Could you check a few things on this model? Use its own coordinates, in mm. Face numbers are marked on the shaded views. Give positions to 0.01 mm unless a question says otherwise; leave off trailing zeros. Loops run counter-clockwise (first coordinate to the right, second up) from the corner with the lowest first, then second, coordinate; pieces in that order, holes last. Notation, with made-up numbers: (58.5, -7) - (89.5, -7) arc R12 ccw to (89.5, -3) - close; hole circle Ø7 at (-21, -13.5). An arc over 180 degrees is marked (long way). Write each question's results on one line, items separated by ' | '. Start each with the question number.
1) I want a section at A-A, the plane x = 6. Write out the boundary of the cut face in (y, z), and give its area (3 significant figures).
2) If we mould it in two halves opening along Z, with no side actions, what happens to the marked faces 1 and 2? For each: +Z half, -Z half, draft (parallel to the pull), parting line (faces both ways), or undercut.
3) I want a section at B-B, the plane z = 66. Write out the boundary of the cut face in (x, y), and give its area (3 significant figures).
4) I want a section at D-D, the plane y = 9. Count the separate pieces of the cut face and the enclosed holes in it, and give its area (3 significant figures).
5) I want a section at C-C, the plane x = 34. Write out the boundary of the cut face in (y, z), and give its area (3 significant figures).
6) I'm going to push flat-ended pins straight in: pin 1 (1 mm diameter, centred on x = 42.5, z = 4, fed in from +Y); pin 2 (3.5 mm diameter, centred on x = -54.46, z = 79.5, fed in from +Y); pin 3 (6.5 mm diameter, centred on x = -54.5, z = -80, fed in from -Y). Where does each tip first touch, or does it pass through?
7) If I drill on probe 1 along Z at (x, y) = (23, 13.75); probe 2 along X at (y, z) = (4.5, 15.5); probe 3 along Y at (x, z) = (-14.5, 73), over which ranges is the centre line in solid material (lowest first)? Write a range as [from, to].
from build123d import *

# Parameters (mm, degrees)
BOSS_EXTRUDE1_DEPTH                                 = 15.0114
CUT_EXTRUDE1_DEPTH                                  = 11.9634
MIRROR2_COPY_1_DEPTH                                = 11.9634
CBORE_SLOT_FOR_3_BINDING_HEAD_MACHINE_S_D           = 4.3688
CBORE_SLOT_FOR_3_BINDING_HEAD_MACHINE_S_CBORE_D     = 7.874
CBORE_SLOT_FOR_3_BINDING_HEAD_MACHINE_S_CBORE_DEPTH = 3.048
MIRROR4_COPY_1_D                                    = 4.3688
MIRROR4_COPY_1_CBORE_D                              = 7.874
MIRROR4_COPY_1_CBORE_DEPTH                          = 3.048
SKETCH10_W                                          = 20.32
SKETCH10_H                                          = 20.32
CUT_EXTRUDE3_DEPTH                                  = 3.048


with BuildPart() as part:
    # Sketch2 → Boss-Extrude1 (new body)
    with BuildSketch(Plane(origin=(0, 0, 0), x_dir=(1, 0, 0), z_dir=(0, 1, 0))):
        with BuildLine():
            Line((56.6928, -85.4964), (-56.6928, -85.4964))
            ThreePointArc((-56.6928, -85.4964), (-59.386876836, -84.380476836), (-60.5028, -81.6864))
            Line((-60.5028, -81.6864), (-60.5028, 81.6864))
            ThreePointArc((-60.5028, 81.6864), (-59.386876836, 84.380476836), (-56.6928, 85.4964))
            Line((-56.6928, 85.4964), (56.6928, 85.4964))
            ThreePointArc((56.6928, 85.4964), (59.386876836, 84.380476836), (60.5028, 81.6864))
            Line((60.5028, 81.6864), (60.5028, -81.6864))
            ThreePointArc((60.5028, -81.6864), (59.386876836, -84.380476836), (56.6928, -85.4964))
        make_face()
    extrude(amount=BOSS_EXTRUDE1_DEPTH)

    # Sketch3 → Cut-Extrude1 (cut)
    with BuildSketch(Plane(origin=(0, 15.0114, 0), x_dir=(1, 0, 0), z_dir=(0, 1, 0))):
        with BuildLine():
            Line((-55.9054, 0), (-55.9054, 71.294481899))
            ThreePointArc((-55.9054, 71.294481899), (-55.361345544, 72.607945544), (-54.047881899, 73.152))
            Line((-54.047881899, 73.152), (-47.553880656, 73.152))
            ThreePointArc((-47.553880656, 73.152), (-44.550315934, 74.249721203), (-42.962410096, 77.0255))
            ThreePointArc((-42.962410096, 77.0255), (-41.374504259, 79.801278797), (-38.370939537, 80.899))
            Line((-38.370939537, 80.899), (0, 80.899))
            Line((0, 80.899), (0, 0))
            Line((0, 0), (-55.9054, 0))
        make_face()
    cut_extrude1 = extrude(amount=-CUT_EXTRUDE1_DEPTH, mode=Mode.SUBTRACT)

    # Mirror1: Cut-Extrude1 across plane
    add(cut_extrude1.mirror(Plane(origin=(0, 0, 0), x_dir=(0, 0, 1), z_dir=(1, 0, 0))), mode=Mode.SUBTRACT)

    # Mirror2: Cut-Extrude1 across plane
    add(cut_extrude1.mirror(Plane.XY), mode=Mode.SUBTRACT)

    # Mirror2 copy 1 sketch → Mirror2 copy 1 (cut)
    with BuildSketch(Plane(origin=(0, 15.0114, 0), x_dir=(-1, 0, 0), z_dir=(0, 1, 0))):
        with BuildLine():
            Line((-55.9054, 0), (-55.9054, 71.294481899))
            ThreePointArc((-55.9054, 71.294481899), (-55.361345544, 72.607945544), (-54.047881899, 73.152))
            Line((-54.047881899, 73.152), (-47.553880656, 73.152))
            ThreePointArc((-47.553880656, 73.152), (-44.550315934, 74.249721203), (-42.962410096, 77.0255))
            ThreePointArc((-42.962410096, 77.0255), (-41.374504259, 79.801278797), (-38.370939537, 80.899))
            Line((-38.370939537, 80.899), (0, 80.899))
            Line((0, 80.899), (0, 0))
            Line((0, 0), (-55.9054, 0))
        make_face()
    extrude(amount=-MIRROR2_COPY_1_DEPTH, mode=Mode.SUBTRACT)

    # CBORE SLOT for #3 Binding Head Machine Screw1 (through all)
    with Locations(Plane(origin=(0, 0, 0), x_dir=(-1, 0, 0), z_dir=(0, -1, 0))):
        with Locations((-54.4576, 79.502)):
            cbore_slot_for_3_binding_head_machine_s = CounterBoreHole(CBORE_SLOT_FOR_3_BINDING_HEAD_MACHINE_S_D / 2, CBORE_SLOT_FOR_3_BINDING_HEAD_MACHINE_S_CBORE_D / 2, CBORE_SLOT_FOR_3_BINDING_HEAD_MACHINE_S_CBORE_DEPTH)

    # Mirror3: CBORE SLOT for #3 Binding Head Machine Screw1 across plane
    add(cbore_slot_for_3_binding_head_machine_s.mirror(Plane(origin=(0, 0, 0), x_dir=(0, 0, 1), z_dir=(1, 0, 0))), mode=Mode.SUBTRACT)

    # Mirror4: CBORE SLOT for #3 Binding Head Machine Screw1 across plane
    add(cbore_slot_for_3_binding_head_machine_s.mirror(Plane.XY), mode=Mode.SUBTRACT)

    # Mirror4 copy 1 (through all)
    with Locations(Plane.XZ):
        with Locations((-54.4576, 79.502)):
            CounterBoreHole(MIRROR4_COPY_1_D / 2, MIRROR4_COPY_1_CBORE_D / 2, MIRROR4_COPY_1_CBORE_DEPTH)

    # Sketch10 → Cut-Extrude3 (cut)
    with BuildSketch(Plane.XZ):
        with Locations((0, 67.66)):
            Rectangle(SKETCH10_W, SKETCH10_H)
    cut_extrude3 = extrude(amount=-CUT_EXTRUDE3_DEPTH, mode=Mode.SUBTRACT)

    # Mirror7: Cut-Extrude3 across plane
    add(cut_extrude3.mirror(Plane.XY), mode=Mode.SUBTRACT)


solid = part.part
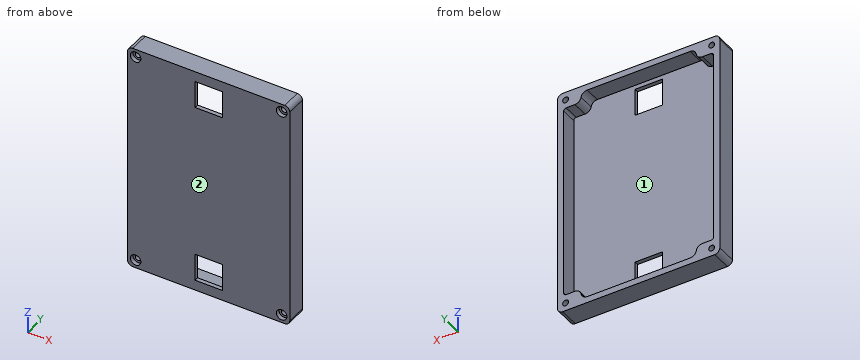
Answers:
1) outline: (0, -85.5) - (15.01, -85.5) - (15.01, -80.9) - (3.05, -80.9) - (3.05, -77.82) - (0, -77.82) - close; (0, -57.5) - (3.05, -57.5) - (3.05, 57.5) - (0, 57.5) - close; (0, 77.82) - (3.05, 77.82) - (3.05, 80.9) - (15.01, 80.9) - (15.01, 85.5) - (0, 85.5) - close | area: 507 mm2
2) face 1: undercut | face 2: draft
3) outline: (-60.5, 0) - (-10.16, 0) - (-10.16, 3.05) - (-55.91, 3.05) - (-55.91, 15.01) - (-60.5, 15.01) - close; (10.16, 0) - (60.5, 0) - (60.5, 15.01) - (55.91, 15.01) - (55.91, 3.05) - (10.16, 3.05) - close | area: 417 mm2
4) separate pieces: 1 | enclosed holes: 5 | area: 2,930 mm2
5) outline: (0, -85.5) - (15.01, -85.5) - (15.01, -80.9) - (3.05, -80.9) - (3.05, 80.9) - (15.01, 80.9) - (15.01, 85.5) - (0, 85.5) - close | area: 631 mm2
6) pin 1: stops at y = 3.05 | pin 2: passes through | pin 3: stops at y = 3.05
7) probe 1: z = [-85.5, -80.9], [80.9, 85.5] | probe 2: x = [-60.5, -55.91], [55.91, 60.5] | probe 3: y = [0, 3.05]
